```python
from build123d import *

# Parameters (mm, degrees)
SKETCH1_W           = 40
SKETCH1_H           = 40
BOSS_EXTRUDE1_DEPTH = 10
SKETCH2_R           = 15
CUT_EXTRUDE1_DEPTH  = 2
FILLET1_R           = 2


with BuildPart() as part:
    # Sketch1 → Boss-Extrude1 (new body)
    with BuildSketch(Plane.YZ):
        Rectangle(SKETCH1_W, SKETCH1_H)
    extrude(amount=BOSS_EXTRUDE1_DEPTH)

    # Sketch2 → Cut-Extrude1 (cut)
    with BuildSketch(Plane.YZ.offset(10)):
        with Locations(Location((3, 0, 0), (0, 0, 270))):
            Circle(SKETCH2_R)
    extrude(amount=-CUT_EXTRUDE1_DEPTH, mode=Mode.SUBTRACT)

    # Fillet1
    fillet1_edges = [part.edges().sort_by_distance(p)[0] for p in [
        (5, 20, -20),
        (5, -20, -20),
        (5, -20, 20),
        (5, 20, 20),
    ]]
    fillet(fillet1_edges, radius=FILLET1_R)


solid = part.part
```
Here's how the part is built. I have some questions about the finished solid (model axes, mm). A direction names the side the tool comes from. Round coordinates to 2 decimals unless told otherwise and drop trailing zeros. Loops run counter-clockwise (first coordinate to the right, second up) from the corner with the lowest first, then second, coordinate; pieces in that order, holes last.
1. Thinking about a two-plate mould opening in Z: for faces 1 (the face through (8, 3, 0)), 2 (the face through (5.07, -19.43, -19.4)), 3 (the face through (0, 0, 0)), which applies, released by +Z, released by -Z, zero draft, split by the parting line, or undercut?
Answers:
face 1: undercut
face 2: released by -Z
face 3: zero draft
2. Suppose I cut it at A-A, the plane z = 0. Please give me the cut outline in (x, y).
Answers:
outline: (0, -20) - (10, -20) - (10, -12) - (8, -12) - (8, 18) - (10, 18) - (10, 20) - (0, 20) - close
3. For faces 4 (the face through (9.014, -11.643, 3.252)), 5 (the face through (5, 0, 20)), which set-ups out of +Z, -Z, +X, -X, +Y, -Y let a thin tool reach every point of the face, with its end or its side?
Answers:
face 4: +X
face 5: +Z, +X, -X, +Y, -Y
4. Suppose I cut it at B-B, the plane y = 1. Please give me the cut outline in (x, z).
Answers:
outline: (0, -20) - (10, -20) - (10, -14.87) - (8, -14.87) - (8, 14.87) - (10, 14.87) - (10, 20) - (0, 20) - close
5. Will this pin go through, and if not, where does the flat tip stop? pin 1 (1.5 mm diameter, centred on y = -2.5, z = -3, fed in from +X).
Answers:
pin 1: stops at x = 8
6. If I drill on probe 1 along Y at (x, z) = (9.3, 0); probe 2 along X at (y, z) = (14, -5); probe 3 along Z at (x, y) = (7.5, 18.5), over which ranges is the centre line in solid material (lowest first)?
Answers:
probe 1: y = -20 to -12, 18 to 20
probe 2: x = 0 to 8
probe 3: z = -19.94 to 19.94
